from build123d import *

# Parameters (mm, degrees)
BLANKSKE_W          = 25
BLANKSKE_H          = 7.3
BLANK_DEPTH         = 4
TOOTHCUTSIM_DEPTH   = 27.349383294
TEETHCUTS_COUNT     = 17
TEETHCUTS_PITCH     = 1.570796325
SKETCH4_W           = 25
SKETCH4_H           = 1.13
BOSS_EXTRUDE1_DEPTH = 2
BOSS_EXTRUDE2_DEPTH = 1
CUT_EXTRUDE1_DEPTH  = 10
SKETCH10_R          = 2
CUT_EXTRUDE3_DEPTH  = 1


with BuildPart() as part:
    # BlankSke → Blank (new body)
    with BuildSketch(Plane.XY):
        with Locations((12.5, 3.65)):
            Rectangle(BLANKSKE_W, BLANKSKE_H)
    extrude(amount=-BLANK_DEPTH)

    # TooCutSkeSim → ToothCutSim (cut, through all)
    with BuildSketch(Plane.XY):
        Polygon((0.222217685, 6.175), (-0.222217685, 6.175), (-0.640929042, 7.3254), (0.640929042, 7.3254), align=None)
    toothcutsim = extrude(amount=-TOOTHCUTSIM_DEPTH, mode=Mode.SUBTRACT)

    # TeethCuts: ToothCutSim ×17
    with Locations(*[(i * TEETHCUTS_PITCH, 0, 0) for i in range(1, TEETHCUTS_COUNT)]):
        add(toothcutsim, mode=Mode.SUBTRACT)

    # Sketch4 → Boss-Extrude1 (add)
    with BuildSketch(Plane.XZ):
        with Locations((12.5, -3.435)):
            Rectangle(SKETCH4_W, SKETCH4_H)
    extrude(amount=BOSS_EXTRUDE1_DEPTH)

    # Sketch7 → Boss-Extrude2 (add)
    with BuildSketch(Plane.XY):
        Polygon((25, 6.175), (24.910523515, 6.175), (24.501057002, 7.3), (24.193629073, 7.3), (23.78416256, 6.175), (23.33972719, 6.175), (22.930260677, 7.3), (22.622832748, 7.3), (22.213366235, 6.175), (21.768930865, 6.175), (21.359464352, 7.3), (21.052036423, 7.3), (20.64256991, 6.175), (20.19813454, 6.175), (19.788668027, 7.3), (19.481240098, 7.3), (19.071773585, 6.175), (18.627338215, 6.175), (18.217871702, 7.3), (17.910443773, 7.3), (17.50097726, 6.175), (17.05654189, 6.175), (16.647075377, 7.3), (16.339647448, 7.3), (15.930180935, 6.175), (15.485745565, 6.175), (15.076279052, 7.3), (14.768851123, 7.3), (14.35938461, 6.175), (13.91494924, 6.175), (13.505482727, 7.3), (13.198054798, 7.3), (12.788588285, 6.175), (12.344152915, 6.175), (11.934686402, 7.3), (11.627258473, 7.3), (11.21779196, 6.175), (10.77335659, 6.175), (10.363890077, 7.3), (10.056462148, 7.3), (9.646995635, 6.175), (9.202560265, 6.175), (8.793093752, 7.3), (8.485665823, 7.3), (8.07619931, 6.175), (7.63176394, 6.175), (7.222297427, 7.3), (6.914869498, 7.3), (6.505402985, 6.175), (6.060967615, 6.175), (5.651501102, 7.3), (5.344073173, 7.3), (4.93460666, 6.175), (4.49017129, 6.175), (4.080704777, 7.3), (3.773276848, 7.3), (3.363810335, 6.175), (2.919374965, 6.175), (2.509908452, 7.3), (2.202480523, 7.3), (1.79301401, 6.175), (1.34857864, 6.175), (0.939112127, 7.3), (0.631684198, 7.3), (0.222217685, 6.175), (0, 6.175), (0, 0), (25, 0), align=None)
    extrude(amount=BOSS_EXTRUDE2_DEPTH)

    # Sketch8 → Cut-Extrude1 (cut)
    with BuildSketch(Plane.XY.offset(1)):
        with BuildLine():
            ThreePointArc((16.617517337, 2), (15.517517337, 3.1), (14.417517337, 2))
            Line((14.417517337, 2), (15.517517337, 2))
            Line((15.517517337, 2), (16.617517337, 2))
        make_face()
        with BuildLine():
            Line((15.517517337, 2), (14.417517337, 2))
            ThreePointArc((14.417517337, 2), (15.517517337, 0.9), (16.617517337, 2))
            Line((16.617517337, 2), (15.517517337, 2))
        make_face()
        with BuildLine():
            ThreePointArc((16.617517337, 2), (15.517517337, 3.1), (14.417517337, 2))
            Line((14.417517337, 2), (15.517517337, 2))
            Line((15.517517337, 2), (16.617517337, 2))
        make_face()
        with BuildLine():
            Line((15.517517337, 2), (14.417517337, 2))
            ThreePointArc((14.417517337, 2), (15.517517337, 0.9), (16.617517337, 2))
            Line((16.617517337, 2), (15.517517337, 2))
        make_face()
        with BuildLine():
            Line((7.705669439, 2), (6.605669439, 2))
            Line((6.605669439, 2), (5.505669439, 2))
            ThreePointArc((5.505669439, 2), (6.605669439, 0.9), (7.705669439, 2))
        make_face()
        with BuildLine():
            Line((5.505669439, 2), (6.605669439, 2))
            Line((6.605669439, 2), (7.705669439, 2))
            ThreePointArc((7.705669439, 2), (6.605669439, 3.1), (5.505669439, 2))
        make_face()
        with BuildLine():
            Line((7.705669439, 2), (6.605669439, 2))
            Line((6.605669439, 2), (5.505669439, 2))
            ThreePointArc((5.505669439, 2), (6.605669439, 0.9), (7.705669439, 2))
        make_face()
        with BuildLine():
            Line((5.505669439, 2), (6.605669439, 2))
            Line((6.605669439, 2), (7.705669439, 2))
            ThreePointArc((7.705669439, 2), (6.605669439, 3.1), (5.505669439, 2))
        make_face()
    extrude(amount=-CUT_EXTRUDE1_DEPTH, mode=Mode.SUBTRACT)

    # Sketch10 → Cut-Extrude3 (cut)
    with BuildSketch(Plane(origin=(0, 0, -4), x_dir=(-1, 0, 0), z_dir=(0, 0, -1))):
        with Locations((-6.605669439, 2)):
            Circle(SKETCH10_R)
    extrude(amount=-CUT_EXTRUDE3_DEPTH, mode=Mode.SUBTRACT)


solid = part.part
Work out the finished part from the listing and answer in its coordinate system (mm). A direction names the side the tool comes from. Coordinates: 2 decimals unless noted, no trailing zeros. Loops run counter-clockwise (first coordinate to the right, second up) from the corner with the lowest first, then second, coordinate; pieces in that order, holes last. Notation, with made-up numbers: M -16.75,7.25 L 15.25,7.25 A23 ccw 15.25,18.25 Z; hole C -36,84.25 d5. An arc over 180 degrees is marked long. Answer in a Markdown table with one row per item. Add a question column.
1. Flat-ended cylindrical pins translate along their axes: P1, Ø0.6, axis at x = 18.5, y = -1, coming from the +Z side; P2, Ø1.9, axis at x = 17, z = -1.5, coming from the -Y side; P3, Ø2, axis at y = 2.5, z = -0.5, coming from the -X side. Find the tip coordinate at first contact, or state that the pin passes through.
2. Find section C-C, the plane z = -2.2. State how many separate pieces and enclosed holes the cut face has, then the cut area to 3 significant figures.
3. The mould has two halves that part along X. Classify faces 4 (the flat face through (12, 0, -1)), 5 (the flat face through (5.7, 1.1, -3)), 6 (the flat face through (0, 3, -2)): pulls with the +X half, pulls with the -X half, needs draft (parallel to the pull), parting line crosses it, or undercut.
4. Find section D-D, the plane y = 0.25. Write down the section's boundary in (x, z), then the cut area to 3 significant figures.
5. Find section B-B, the plane y = 3.5. Write down the section's boundary in (x, z), then the cut area to 3 significant figures.
6. Consider L1, parallel to X at y = 2.25, z = -2.45; L2, parallel to Z at x = 1.5, y = -1.25; L3, parallel to Y at x = 20.5, z = -0.2 (3 decimals). Determine where each line is inside the solid, lowest interval first.
7. A tool of negligible diameter and unlimited length cuts with its end or side. For faces 1 (the flat face through (12, 4, 1)), 2 (the flat face through (12, -1, -2.87)), 3 (the cylindrical face through (5.683, 0.226, -3.507)), from which of +Z, -Z, +X, -X, +Y, -Y can it reach the whole face along a straight path? Write none if from no direction.
8. Find section A-A, the plane y = 2. Write down the section's boundary in (x, z).
Reported:
| question | item | result |
|---|---|---|
| 1 | P1 | stops at z = -2.87 |
| 1 | P2 | stops at y = 0 |
| 1 | P3 | stops at x = 0 |
| 2 | separate pieces | 1 |
| 2 | enclosed holes | 2 |
| 2 | area | 160 mm^2 |
| 3 | face 4 | needs draft |
| 3 | face 5 | undercut |
| 3 | face 6 | pulls with the -X half |
| 4 | outline | M 0,-4 L 5.64,-4 L 5.64,-3 L 7.57,-3 L 7.57,-4 L 25,-4 L 25,1 L 0,1 Z |
| 4 | area | 123 mm^2 |
| 5 | outline | M 0,-4 L 5.28,-4 L 5.28,-3 L 7.93,-3 L 7.93,-4 L 25,-4 L 25,1 L 0,1 Z |
| 5 | area | 122 mm^2 |
| 6 | L1 | x = 0 to 5.53, 7.68 to 14.45, 16.59 to 25 |
| 6 | L2 | z = -4 to -2.87 |
| 6 | L3 | y = 0 to 6.175 |
| 7 | face 1 | +Z, +X, -X, +Y, -Y |
| 7 | face 2 | +Z, +X, -X, -Y |
| 7 | face 3 | -Z |
| 8 | outline | M 0,-4 L 4.61,-4 L 4.61,-3 L 5.51,-3 L 5.51,1 L 0,1 Z; M 7.71,-3 L 8.61,-3 L 8.61,-4 L 14.42,-4 L 14.42,1 L 7.71,1 Z; M 16.62,-4 L 25,-4 L 25,1 L 16.62,1 Z |
